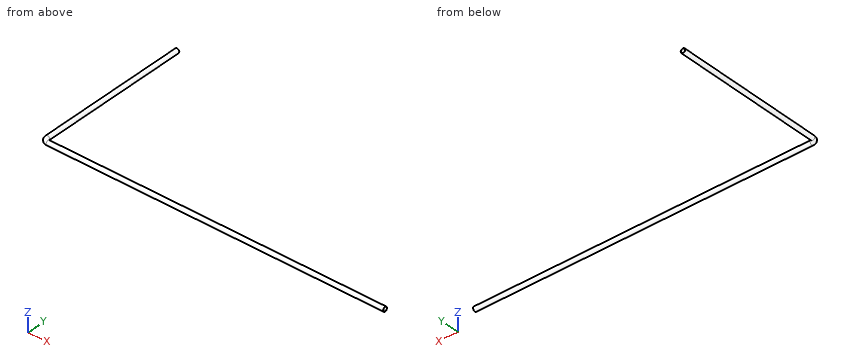
from build123d import *

# Parameters (mm, degrees)
SWEEP_THIN1_PROFILE_R   = 15
SWEEP_THIN1_PROFILE_R_2 = 14


with BuildPart() as part:
    # Sweep-Thin1: sweep along a curve in space
    with BuildLine() as sweep_thin1_path:
        Line((-34220.216064675, -16256.702563295, 40211.577712625), (-34220.216064675, -17268.210932222, 40211.577712625))
        ThreePointArc((-34190.216064675, -17298.210932222, 40211.577712625), (-34211.429268111, -17289.424135658, 40211.577712625), (-34220.216064675, -17268.210932222, 40211.577712625))
        Line((-34190.216064675, -17298.210932222, 40211.577712625), (-31937.449283249, -17298.210932222, 40211.577712625))
    # Sweep-Thin1 profile (on start of the path) → Sweep-Thin1 (sweep)
    with BuildSketch(Plane(origin=(-34220.216064675, -16256.702563295, 40211.577712625), x_dir=(0, 0, -1), z_dir=(0, -1, 0))):
        Circle(SWEEP_THIN1_PROFILE_R)
        Circle(SWEEP_THIN1_PROFILE_R_2, mode=Mode.SUBTRACT)
    sweep(path=sweep_thin1_path.line)


solid = part.part
Read the model definition and answer for the solid it produces. Units are mm, in the model's axes. Round coordinates to 2 decimals unless told otherwise and drop trailing zeros. Order: outer loops, then holes, each group sorted by start corner. A loop starts at its lowest first (then second) coordinate and runs counter-clockwise, first axis right, second up.
1) Flat-ended cylindrical pins translate along their axes: pin 1 (5 mm diameter, centred on x = -33678, z = 40215, fed in from +Y); pin 2 (1.5 mm diameter, centred on y = -16380, z = 40215, fed in from -X); pin 3 (1.5 mm diameter, centred on x = -32542, z = 40205.5, fed in from +Y). Find the tip coordinate at first contact, or state that the pin passes through.
2) Straight lines are drawn through the part: L1, parallel to Y at x = -33273.5, z = 40208; L2, parallel to X at y = -16838.5, z = 40208; L3, parallel to Y at x = -32204, z = 40210.5. For each, find the intervals that lie inside material, in ascending order.
3) The part is cut by section A-A on y = -17069. Write down the section's boundary in (x, z), plus the area to 3 significant figures.
Resolved:
1. pin 1: stops at y = -17283.24
1. pin 2: stops at x = -34234.98
1. pin 3: stops at y = -17284.19
2. L1: y = -17312.78 to -17311.75, -17284.68 to -17283.64
2. L2: x = -34234.78 to -34233.75, -34206.68 to -34205.65
2. L3: y = -17313.17 to -17312.17, -17284.25 to -17283.25
3. outline: circle Ø30 at (-34220.22, 40211.58); hole circle Ø28 at (-34220.22, 40211.58)
3. area: 91.1 mm2
